The figure shows three views and two pictorial views of one solid part (mm, origin at its lowest corner). Answer the questions. A direction names the side the tool comes from. Round coordinates to 2 decimals unless told otherwise and drop trailing zeros. Order: outer loops, then holes, each group sorted by start corner. A loop starts at its lowest first (then second) coordinate and runs counter-clockwise, first axis right, second up. Notation, with made-up numbers: (37, 45) - (87, 45) arc R22 cw to (87, 72) - close; hole circle Ø9 at (12, 72). An arc over 180 degrees is marked (long way). Write item = value, one per line.
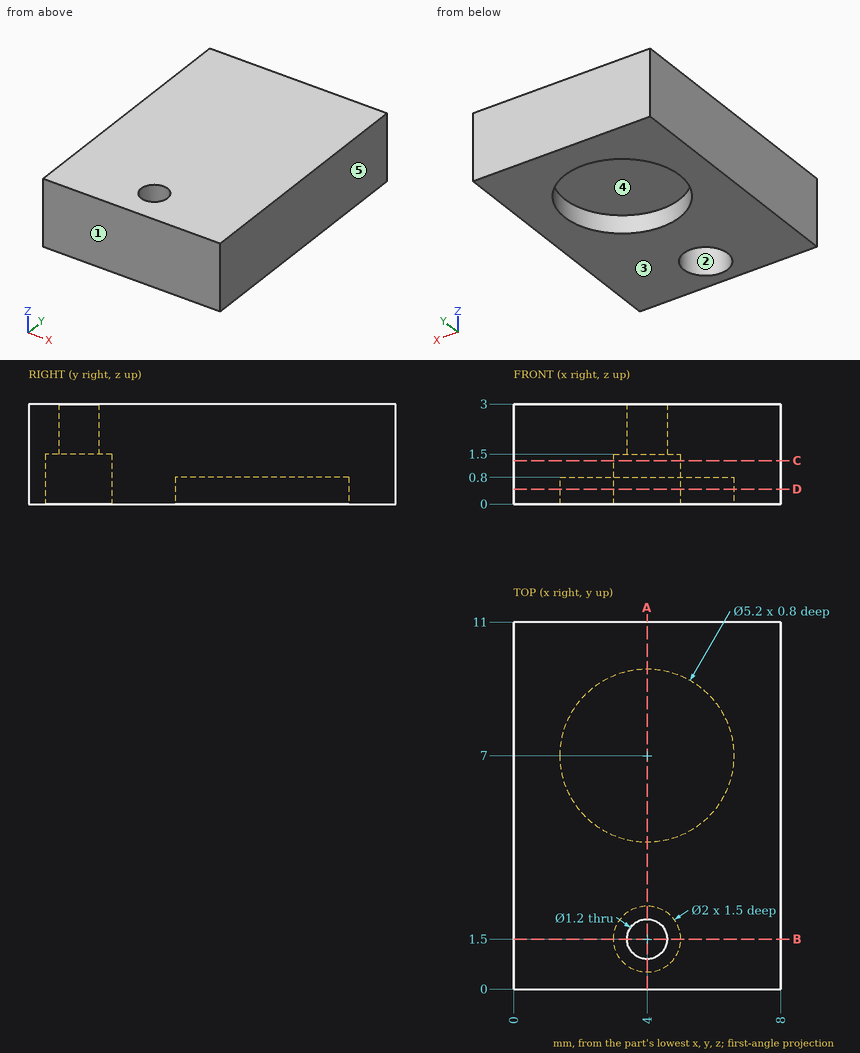
Q1. Determine the mould class of the marked faces 1, 2 and 3 for opening direction Y: released by +Y, released by -Y, zero draft, split by the parting line, or undercut.
Model answer:
face_1 = released by -Y
face_2 = undercut
face_3 = zero draft
Q2. Section A-A on x = 4 is taken. Determine the outline of the cut face in (y, z), then the cut area to 3 significant figures.
Model answer:
outline = (0, 0) - (0.5, 0) - (0.5, 1.5) - (0.9, 1.5) - (0.9, 3) - (0, 3) - close; (2.1, 1.5) - (2.5, 1.5) - (2.5, 0) - (4.4, 0) - (4.4, 0.8) - (9.6, 0.8) - (9.6, 0) - (11, 0) - (11, 3) - (2.1, 3) - close
area = 24.0 mm^2
Q3. Section D-D on z = 0.45 is taken. Determine the outline of the cut face in (x, y), then the cut area to 3 significant figures.
Model answer:
outline = (0, 0) - (8, 0) - (8, 11) - (0, 11) - close; hole circle Ø5.2 at (4, 7); hole circle Ø2 at (4, 1.5)
area = 63.6 mm^2
Q4. Section C-C on z = 1.3 is taken. Determine the outline of the cut face in (x, y).
Model answer:
outline = (0, 0) - (8, 0) - (8, 11) - (0, 11) - close; hole circle Ø2 at (4, 1.5)
Q5. Section B-B on y = 1.5 is taken. Determine the outline of the cut face in (x, z).
Model answer:
outline = (0, 0) - (3, 0) - (3, 1.5) - (3.4, 1.5) - (3.4, 3) - (0, 3) - close; (4.6, 1.5) - (5, 1.5) - (5, 0) - (8, 0) - (8, 3) - (4.6, 3) - close
Q6. For the marked faces 4 and 5, determine the directions among +Z, -Z, +X, -X, +Y, -Y from which every point of the face is accessible in a straight line to the end or side of a thin tool.
Model answer:
face_4 = -Z
face_5 = +Z, -Z, +X, +Y, -Y
Q7. A flat-ended cylindrical pin translates along its axis: P1, Ø1.9, axis at x = 4, y = 1.5, coming from the +Z side. Find the tip coordinate at first contact, or state that the pin passes through.
Model answer:
P1 = 3
Q8. Find the intervals of material crossed by line 1 (Y direction, x = 4, z = 0.65); line 2 (Y direction, x = 3.5, z = 0.75); line 3 (Z direction, x = 5.75, y = 5.5), in increasing order. Write a range as from..to.
Model answer:
line_1 = 0..0.5, 2.5..4.4, 9.6..11
line_2 = 0..0.63, 2.37..4.45, 9.55..11
line_3 = 0.8..3
